```python
from build123d import *

# Parameters (mm, degrees)
EXTRUDE1_DEPTH     = 21.59
SKETCH3_R          = 2.54
CUT_EXTRUDE1_DEPTH = 21.59


with BuildPart() as part:
    # Sketch2 → Extrude1 (new body)
    with BuildSketch(Plane.XY):
        with BuildLine():
            Line((137.16, -6013.450000001), (-603.25, -6013.450000001))
            Line((-603.25, -6013.450000001), (-603.25, -5867.400000001))
            Line((-603.25, -5867.400000001), (-155.878238141, -5867.400000001))
            ThreePointArc((-155.878238141, -5867.400000001), (-141.328560309, -5864.951302064), (-128.38193157, -5857.875))
            ThreePointArc((-128.38193157, -5857.875), (-115.435302831, -5850.798697937), (-100.885625, -5848.35))
            Line((-100.885625, -5848.35), (-50.085625, -5848.35))
            ThreePointArc((-50.085625, -5848.35), (-35.535947169, -5850.798697937), (-22.58931843, -5857.875))
            ThreePointArc((-22.58931843, -5857.875), (-9.642689691, -5864.951302063), (4.906988141, -5867.400000001))
            Line((4.906988141, -5867.400000001), (137.16, -5867.400000001))
            Line((137.16, -5867.400000001), (137.16, -6013.450000001))
        make_face()
    extrude(amount=-EXTRUDE1_DEPTH)

    # Sketch3 → Cut-Extrude1 (cut)
    with BuildSketch(Plane.XY):
        with Locations((-333.454375, -5994.4)):
            Circle(SKETCH3_R)
        with Locations((-132.635625, -5994.4)):
            Circle(SKETCH3_R)
        with Locations((-132.635625, -5894.07)):
            Circle(SKETCH3_R)
        with Locations((-333.454375, -5894.07)):
            Circle(SKETCH3_R)
        with BuildLine():
            Line((-104.060625, -5892.8), (-104.060625, -5969))
            ThreePointArc((-104.060625, -5969), (-103.13068903, -5971.24506403), (-100.885625, -5972.175))
            Line((-100.885625, -5972.175), (-50.085625, -5972.175))
            ThreePointArc((-50.085625, -5972.175), (-47.84056097, -5971.24506403), (-46.910625, -5969))
            Line((-46.910625, -5969), (-46.910625, -5892.8))
            Line((-46.910625, -5892.8), (-50.085625, -5889.625))
            Line((-50.085625, -5889.625), (-100.885625, -5889.625))
            ThreePointArc((-100.885625, -5889.625), (-103.13068903, -5890.55493597), (-104.060625, -5892.8))
        make_face()
    extrude(amount=-CUT_EXTRUDE1_DEPTH, mode=Mode.SUBTRACT)


solid = part.part
```
Could you check a few things on this model? Use its own coordinates, in mm. A direction names the side the tool comes from. Give positions to 0.01 mm unless a question says otherwise; leave off trailing zeros. Loops run counter-clockwise (first coordinate to the right, second up) from the corner with the lowest first, then second, coordinate; pieces in that order, holes last. Notation, with made-up numbers: (51, 68) - (60, 68) arc R27 cw to (60, 95) - close; hole circle Ø6 at (-25.5, 35.25). An arc over 180 degrees is marked (long way). Answer in a Markdown table with one row per item. Add a question column.
Q1. If we section it at A-A (y = -5953.5): List the corners of the cut face in (x, z) for me, plus the area to 3 significant figures.
Q2. Please list where these lines run through material, in increasing order: L1, parallel to X at y = -5994.4, z = -8.5; L2, parallel to X at y = -5894.07, z = -11.5; L3, parallel to X at y = -5894.5, z = -12. Write a range as from..to.
Q3. For pin 1 (6.5 mm diameter, centred on x = -427.5, z = -9.5, fed in from +Y); pin 2 (8 mm diameter, centred on x = -8.5, z = -17, fed in from +Y), each with a flat end and sliding along its axis, tell me the tip position at first contact or that it passes through.
Q4. If we section it at C-C (x = -170.5): List the corners of the cut face in (y, z) for me.
Q5. If we section it at B-B (z = -12.75): List the corners of the cut face in (x, y) for me (3 decimals).
Q6. Which directions (+Z, -Z, +X, -X, +Y, -Y) give clear straight access to the entire face, cutting with the end or side of a thin tool? Please do faces 1 (the face through (137.16, -5939, -11)), 2 (the face through (-75, -5889.625, -11)), 3 (the face through (70, -5867.4, -11)), 4 (the face through (-383, -5867.4, -11)).
Q7. We'd pull the mould along Y, two halves only. Please class faces 5 (the face through (-228, -5930, 0)), 6 (the face through (-104.061, -5930, -11)), 7 (the face through (-76, -5848.35, -11)): +Y half, -Y half, draft (parallel to the pull), parting line (faces both ways), or undercut.
The answers:
| question | item | result |
|---|---|---|
| 1 | outline | (-603.25, -21.59) - (-104.06, -21.59) - (-104.06, 0) - (-603.25, 0) - close; (-46.91, -21.59) - (137.16, -21.59) - (137.16, 0) - (-46.91, 0) - close |
| 1 | area | 14,800 mm^2 |
| 2 | L1 | x = -603.25..-335.99, -330.91..-135.18, -130.1..137.16 |
| 2 | L2 | x = -603.25..-335.99, -330.91..-135.18, -130.1..-104.06, -46.91..137.16 |
| 2 | L3 | x = -603.25..-335.96, -330.95..-135.14, -130.13..-104.06, -46.91..137.16 |
| 3 | pin 1 | stops at y = -5867.4 |
| 3 | pin 2 | stops at y = -5863.85 |
| 4 | outline | (-6013.45, -21.59) - (-5867.4, -21.59) - (-5867.4, 0) - (-6013.45, 0) - close |
| 5 | outline | (-603.25, -6013.45) - (137.16, -6013.45) - (137.16, -5867.4) - (4.907, -5867.4) arc R44.45 cw to (-22.589, -5857.875) arc R44.45 ccw to (-50.086, -5848.35) - (-100.886, -5848.35) arc R44.45 ccw to (-128.382, -5857.875) arc R44.45 cw to (-155.878, -5867.4) - (-603.25, -5867.4) - close; hole circle Ø5.08 at (-333.454, -5994.4); hole circle Ø5.08 at (-333.454, -5894.07); hole circle Ø5.08 at (-132.636, -5994.4); hole circle Ø5.08 at (-132.636, -5894.07); hole (-104.061, -5969) arc R3.175 ccw to (-100.886, -5972.175) - (-50.086, -5972.175) arc R3.175 ccw to (-46.911, -5969) - (-46.911, -5892.8) - (-50.086, -5889.625) - (-100.886, -5889.625) arc R3.175 ccw to (-104.061, -5892.8) - close |
| 6 | face 1 | +Z, -Z, +X, +Y, -Y |
| 6 | face 2 | +Z, -Z |
| 6 | face 3 | +Z, -Z, +X, +Y |
| 6 | face 4 | +Z, -Z, -X, +Y |
| 7 | face 5 | draft |
| 7 | face 6 | undercut |
| 7 | face 7 | +Y half |
